```python
from build123d import *

# Parameters (mm, degrees)
SKETCH1_R             = 21
SKETCH1_R_2           = 16
BOSS_EXTRUDE1_DEPTH   = 10
SKETCH1_R_3           = 12.5
SKETCH1_R_4           = 6.25
BOSS_EXTRUDE1_2_DEPTH = 10
BOSS_EXTRUDE4_DEPTH   = 6
BOSS_EXTRUDE6_DEPTH   = 6
BOSS_EXTRUDE7_DEPTH   = 6
CUT_EXTRUDE1_START    = 6
CUT_EXTRUDE1_DEPTH    = 132.802456026
CUT_EXTRUDE3_START    = -6
CUT_EXTRUDE3_DEPTH    = 132.802456026


with BuildPart() as part:
    # Sketch1 → Boss-Extrude1 (new, symmetric)
    with BuildSketch(Plane.XY):
        Circle(SKETCH1_R)
        Circle(SKETCH1_R_2, mode=Mode.SUBTRACT)
    extrude(amount=BOSS_EXTRUDE1_DEPTH, both=True)



with BuildPart() as body_2:
    # Sketch1 → Boss-Extrude1 2 (new, symmetric)
    with BuildSketch(Plane.XY):
        with Locations((0, 120)):
            Circle(SKETCH1_R_3)
        with Locations((0, 120)):
            Circle(SKETCH1_R_4, mode=Mode.SUBTRACT)
    extrude(amount=BOSS_EXTRUDE1_2_DEPTH, both=True)


with BuildPart() as part_1:
    add(part.part)

    add(body_2.part)  # Boss-Extrude4 merges body 2
    # Sketch1_5 → Boss-Extrude4 (add, symmetric)
    with BuildSketch(Plane.XY):
        with BuildLine():
            ThreePointArc((8, 110.395313644), (0, 107.5), (-8, 110.395313644))
            Line((-8, 110.395313644), (-8, 75.395313644))
            ThreePointArc((-8, 75.395313644), (-10.96842855, 40.709642053), (-19.787382488, 7.032744434))
            ThreePointArc((-19.787382488, 7.032744434), (0, 21), (19.787382488, 7.032744434))
            ThreePointArc((19.787382488, 7.032744434), (10.96842855, 40.709642053), (8, 75.395313644))
            Line((8, 75.395313644), (8, 110.395313644))
        make_face()
    extrude(amount=BOSS_EXTRUDE4_DEPTH, both=True)

    # Sketch1_8 → Boss-Extrude6 (add, symmetric)
    with BuildSketch(Plane.XY):
        with BuildLine():
            ThreePointArc((16.961079982, -12.382316659), (-0.033074929, -20.999973954), (-17, -12.328828006))
            Line((-17, -12.328828006), (-17, -24.328828006))
            Line((-17, -24.328828006), (17, -24.328828006))
            Line((17, -24.328828006), (16.961079982, -12.382316659))
        make_face()
    extrude(amount=BOSS_EXTRUDE6_DEPTH, both=True)

    # Sketch1_9 → Boss-Extrude7 (add, symmetric)
    with BuildSketch(Plane.XY):
        with BuildLine():
            Line((-6.25, 135.825317547), (-6.25, 130.825317547))
            ThreePointArc((-6.25, 130.825317547), (0, 132.5), (6.25, 130.825317547))
            Line((6.25, 130.825317547), (6.25, 135.825317547))
            Line((6.25, 135.825317547), (-6.25, 135.825317547))
        make_face()
    extrude(amount=BOSS_EXTRUDE7_DEPTH, both=True)

    # Sketch4 → Cut-Extrude1 (cut, through all)
    with BuildSketch(Plane(origin=(0, 0, 0), x_dir=(0, 0, -1), z_dir=(1, 0, 0)).offset(CUT_EXTRUDE1_START)):
        with BuildLine():
            Line((4, 100), (4, 38))
            ThreePointArc((4, 38), (0, 34), (-4, 38))
            Line((-4, 38), (-4, 100))
            ThreePointArc((-4, 100), (0, 104), (4, 100))
        make_face()
    extrude(amount=CUT_EXTRUDE1_DEPTH, mode=Mode.SUBTRACT)

    # Sketch4_3 → Cut-Extrude3 (cut, through all)
    with BuildSketch(Plane(origin=(0, 0, 0), x_dir=(0, 0, -1), z_dir=(1, 0, 0)).offset(CUT_EXTRUDE3_START)):
        with BuildLine():
            Line((4, 100), (4, 38))
            ThreePointArc((4, 38), (0, 34), (-4, 38))
            Line((-4, 38), (-4, 100))
            ThreePointArc((-4, 100), (0, 104), (4, 100))
        make_face()
    extrude(amount=-CUT_EXTRUDE3_DEPTH, mode=Mode.SUBTRACT)


solid = part_1.part
```
Design review of the part built by this model. Coordinates are the model's own, in mm. A direction names the side the tool comes from. Coordinates: 2 decimals unless noted, no trailing zeros. Write each loop counter-clockwise with the first axis right and the second up, starting at its lowest first coordinate (ties: lowest second). Pieces come first, ordered by that corner, then holes.
1) Machinability: for faces 5 (the flat face through (-17, -18, 0)), 6 (the flat face through (6.25, 133, 0)), 7 (the flat face through (-8, 97, 5)), 8 (the flat face through (-7, 62, 4)), 9 (the flat face through (0, -22, -6)), which of the approach directions +Z, -Z, +X, -X, +Y, -Y give a long, thin tool a straight path to every point of the face, cutting with its end or side? Answer none if there is none.
2) Add section C-C (z = 8.5). Write out the cut boundary in (x, y), plus the area to 3 significant figures.
3) Add section A-A (y = 0). Write out the cut boundary in (x, z), plus the area to 3 significant figures.
4) Add section B-B (x = -3.5). Write out the cut boundary in (y, z), plus the area to 3 significant figures.
5) Add section D-D (z = 0). Write out the cut boundary in (x, y), plus the area to 3 significant figures.
6) Mouldability with a two-part tool opening along Z and no side actions: class faces 1 (the flat face through (8, 97, 5)), 2 (the flat face through (7, 62, 4)), 3 (the flat face through (0, 134, -6)), 4 (the flat face through (0, -22, 6)) as +Z half, -Z half, draft (parallel to the pull), parting line (faces both ways), or undercut.
7) To check wall thickness, follow L1, parallel to Y at x = 0, z = 3.25; L2, parallel to Y at x = -3.5, z = -8.25; L3, parallel to Y at x = 1, z = 7.5. State the ranges of each line that lie inside material, in increasing order.
8) Insertion check: pin 1 (8 mm diameter, centred on x = 4.5, y = 108, fed in from +Z); pin 2 (5.5 mm diameter, centred on y = 132, z = -0.5, fed in from +X); pin 3 (2.5 mm diameter, centred on x = 8, y = 79, fed in from -Z); pin 4 (4 mm diameter, centred on y = 65.5, z = -1, fed in from -X). Each pin has a flat end and moves straight along its axis. Give the tip position at first contact, or say it passes through.
Check result:
1. face 5: +Z, -Z, -X, -Y
1. face 6: +Z, -Z, +X, +Y
1. face 7: +Z, -Z, -X
1. face 8: -X
1. face 9: -Z, -Y
2. outline: circle Ø42 at (0, 0); circle Ø25 at (0, 120); hole circle Ø32 at (0, 0); hole circle Ø12.5 at (0, 120)
2. area: 949 mm2
3. outline: (-21, -10) - (-16, -10) - (-16, 10) - (-21, 10) - close; (16, -10) - (21, -10) - (21, 10) - (16, 10) - close
3. area: 200 mm2
4. outline: (-24.33, -6) - (-20.71, -6) - (-20.71, -10) - (-15.61, -10) - (-15.61, 10) - (-20.71, 10) - (-20.71, 6) - (-24.33, 6) - close; (15.61, -10) - (20.71, -10) - (20.71, -6) - (108, -6) - (108, -10) - (114.82, -10) - (114.82, 10) - (108, 10) - (108, 6) - (20.71, 6) - (20.71, 10) - (15.61, 10) - close; (125.18, -10) - (132, -10) - (132, -6) - (135.83, -6) - (135.83, 6) - (132, 6) - (132, 10) - (125.18, 10) - close
4. area: 1,610 mm2
5. outline: (-19.79, 7.03) arc R21 ccw to (-17, -12.33) - (-17, -24.33) - (17, -24.33) - (16.96, -12.38) arc R21 ccw to (19.79, 7.03) arc R204.13 cw to (12.24, 34) - (6, 34) - (6, 104) - (8, 104) - (8, 110.4) arc R12.5 ccw to (6.25, 130.83) - (6.25, 135.83) - (-6.25, 135.83) - (-6.25, 130.83) arc R12.5 ccw to (-8, 110.4) - (-8, 104) - (-6, 104) - (-6, 34) - (-12.24, 34) arc R204.13 cw to start; hole circle Ø32 at (0, 0); hole circle Ø12.5 at (0, 120)
5. area: 2,550 mm2
6. face 1: draft
6. face 2: undercut
6. face 3: -Z half
6. face 4: +Z half
7. L1: y = -24.33 to -16, 16 to 113.75, 126.25 to 135.83
7. L2: y = -20.71 to -15.61, 15.61 to 20.71, 108 to 114.82, 125.18 to 132
7. L3: y = -20.98 to -15.97, 15.97 to 20.98, 107.54 to 113.83, 126.17 to 132.46
8. pin 1: stops at z = 10
8. pin 2: stops at x = 8.41
8. pin 3: stops at z = -6
8. pin 4: stops at x = -6
